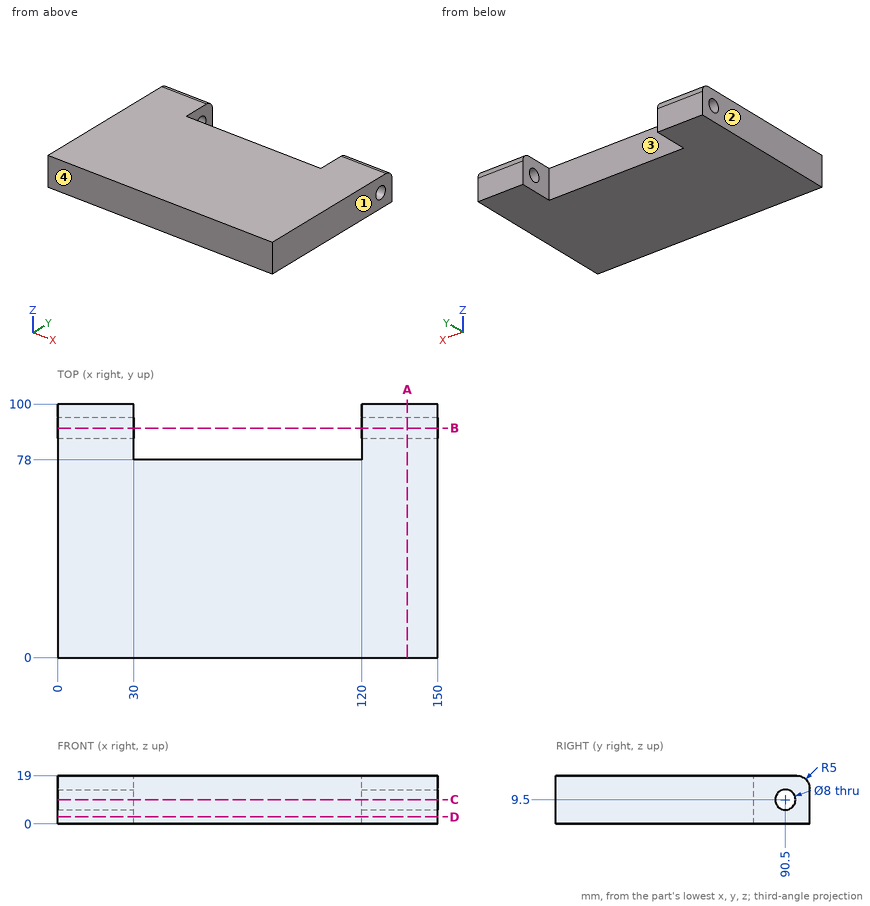
Here's the drawing with two shaded views (mm, measured from the low corner). I have some questions. Give positions to 0.01 mm unless a question says otherwise; leave off trailing zeros. Loops run counter-clockwise (first coordinate to the right, second up) from the corner with the lowest first, then second, coordinate; pieces in that order, holes last. Notation, with made-up numbers: (6.25, 82.5) -> (26.25, 82.5) arc R22 cw to (26.25, 120.5) -> close; hole circle Ø3 at (79, 83). An arc over 180 degrees is marked (long way). One line per item, written item: value.
Q1. Suppose I cut it at A-A on x = 138. Please give me the cut outline in (y, z), then the cut area to 3 significant figures.
Answers follow:
outline: (0, 0) -> (100, 0) -> (100, 14) arc R5 ccw to (95, 19) -> (0, 19) -> close; hole circle Ø8 at (90.5, 9.5)
area: 1,840 mm^2
Q2. Suppose I cut it at D-D on z = 2.75. Please give me the cut outline in (x, y), then the cut area to 3 significant figures.
Answers follow:
outline: (0, 0) -> (150, 0) -> (150, 100) -> (120, 100) -> (120, 78) -> (30, 78) -> (30, 100) -> (0, 100) -> close
area: 13,000 mm^2
Q3. Suppose I cut it at B-B on y = 90.5. Please give me the cut outline in (x, z).
Answers follow:
outline: (0, 0) -> (30, 0) -> (30, 5.5) -> (0, 5.5) -> close; (0, 13.5) -> (30, 13.5) -> (30, 19) -> (0, 19) -> close; (120, 0) -> (150, 0) -> (150, 5.5) -> (120, 5.5) -> close; (120, 13.5) -> (150, 13.5) -> (150, 19) -> (120, 19) -> close
Q4. Suppose I cut it at C-C on z = 9.5. Please give me the cut outline in (x, y), then the cut area to 3 significant figures.
Answers follow:
outline: (0, 0) -> (150, 0) -> (150, 86.5) -> (120, 86.5) -> (120, 78) -> (30, 78) -> (30, 86.5) -> (0, 86.5) -> close; (0, 94.5) -> (30, 94.5) -> (30, 100) -> (0, 100) -> close; (120, 94.5) -> (150, 94.5) -> (150, 100) -> (120, 100) -> close
area: 12,500 mm^2
Q5. I'm going to push a flat-ended pin straight in: pin 1 Ø6 at (x, z) = (104, 15) entering from +Y. Where does the tip first touch, or does it pass through?
Answers follow:
pin 1: y = 78
Q6. If I drill on line 1 along Z through (x, y) = (143.5, 90.5); line 2 along X through (y, z) = (81.5, 12); line 3 along Y through (x, z) = (113, 1), over which ranges is the centre line in solid material (lowest first)?
Answers follow:
line 1: 0 to 5.5, 13.5 to 19
line 2: 0 to 30, 120 to 150
line 3: 0 to 78
Q7. We'd pull the mould along X, two halves only. Please class the marked faces 1, 2, 3 and 4: pulls with the +X half, pulls with the -X half, needs draft (parallel to the pull), parting line crosses it, or undercut.
Answers follow:
face 1: pulls with the +X half
face 2: pulls with the -X half
face 3: undercut
face 4: needs draft
